For this review, take the finished solid that the model builds, in its own axes (mm). A direction names the side the tool comes from. Give positions to 0.01 mm unless a question says otherwise; leave off trailing zeros. Order: outer loops, then holes, each group sorted by start corner. A loop starts at its lowest first (then second) coordinate and runs counter-clockwise, first axis right, second up. Notation, with made-up numbers: (75.5, 12.25) - (96.5, 12.25) arc R19 ccw to (96.5, 19.25) - close; hole circle Ø9 at (7, 27.5). An arc over 180 degrees is marked (long way). One line per item, written item: value.
```python
from build123d import *

# Parameters (mm, degrees)
SKETCH1_W           = 50.8
SKETCH1_H           = 50.8
SKETCH1_W_2         = 44.45
SKETCH1_H_2         = 44.45
EXTRUDE1_DEPTH      = 1117.6
EXTRUDE1_DEPTH_BACK = 50.8
SKETCH3_R           = 6.35
CUT_EXTRUDE2_DEPTH  = 51.8


with BuildPart() as part:
    # Sketch1 → Extrude1 (new body, two sides)
    with BuildSketch(Plane.XY) as extrude1_sk:
        with Locations((-514.35, 304.8)):
            Rectangle(SKETCH1_W, SKETCH1_H)
        with Locations((-514.35, 304.8)):
            Rectangle(SKETCH1_W_2, SKETCH1_H_2, mode=Mode.SUBTRACT)
    extrude(amount=EXTRUDE1_DEPTH)
    extrude(extrude1_sk.sketch, amount=-EXTRUDE1_DEPTH_BACK)

    # Sketch3 → Cut-Extrude2 (cut, through all)
    with BuildSketch(Plane(origin=(0, 330.2, 0), x_dir=(1, 0, 0), z_dir=(0, 1, 0))):
        with Locations((-514.35, -1092.2)):
            Circle(SKETCH3_R)
        with Locations((-514.35, -958.85)):
            Circle(SKETCH3_R)
        with Locations((-514.35, -590.55)):
            Circle(SKETCH3_R)
        with Locations((-514.35, -222.25)):
            Circle(SKETCH3_R)
    extrude(amount=-CUT_EXTRUDE2_DEPTH, mode=Mode.SUBTRACT)


solid = part.part
```
(1) Machinability: for faces 1 (the face through (-536.575, 304, 542)), 2 (the face through (-515, 279.4, 542)), which of the approach directions +Z, -Z, +X, -X, +Y, -Y give a long, thin tool a straight path to every point of the face, cutting with its end or side? Answer none if there is none.
Answers below:
face 1: +Z, -Z
face 2: +Z, -Z, +X, -X, -Y
(2) Wall thickness on line 1 (Z direction, x = -514.35, y = 280.3); line 2 (Y direction, x = -496, z = 138.5) (3 decimals); line 3 (X direction, y = 281, z = 958): over which ranges is each line inside the solid? List them lowest first. Write a range as from..to.
Answers below:
line 1: z = -50.8..215.9, 228.6..584.2, 596.9..952.5, 965.2..1085.85, 1098.55..1117.6
line 2: y = 279.4..282.575, 327.025..330.2
line 3: x = -539.75..-520.64, -508.06..-488.95
(3) For P1, Ø11.5, axis at x = -514.35, z = 590.55, coming from the -Y side, flat-tipped, find the tip position at first contact; note if it passes through.
Answers below:
P1: passes through
(4) Take a section at A-A (z = 435). Write out the cut boundary in (x, y) (3 decimals), then the cut area to 3 significant figures.
Answers below:
outline: (-539.75, 279.4) - (-488.95, 279.4) - (-488.95, 330.2) - (-539.75, 330.2) - close; hole (-536.575, 282.575) - (-492.125, 282.575) - (-492.125, 327.025) - (-536.575, 327.025) - close
area: 605 mm^2
(5) Draft analysis for pull direction X (two halves, no side actions). For faces 3 (the face through (-492.125, 304, 542)), 4 (the face through (-537, 305, 1117.6)), 5 (the face through (-488.95, 304, 542)), state which applies: pulls with the +X half, pulls with the -X half, needs draft (parallel to the pull), parting line crosses it, or undercut.
Answers below:
face 3: undercut
face 4: needs draft
face 5: pulls with the +X half
(6) Take a section at B-B (y = 319). Write out the cut boundary in (x, z) (3 decimals), then the cut area to 3 significant figures.
Answers below:
outline: (-539.75, -50.8) - (-536.575, -50.8) - (-536.575, 1117.6) - (-539.75, 1117.6) - close; (-492.125, -50.8) - (-488.95, -50.8) - (-488.95, 1117.6) - (-492.125, 1117.6) - close
area: 7,420 mm^2
(7) Take a section at C-C (x = -500). Write out the cut boundary in (y, z) (3 decimals), then the cut area to 3 significant figures.
Answers below:
outline: (279.4, -50.8) - (282.575, -50.8) - (282.575, 1117.6) - (279.4, 1117.6) - close; (327.025, -50.8) - (330.2, -50.8) - (330.2, 1117.6) - (327.025, 1117.6) - close
area: 7,420 mm^2
